The model under review builds one solid part; all positions refer to its coordinate system, in mm. A direction names the side the tool comes from. Round coordinates to 2 decimals unless told otherwise and drop trailing zeros. Loops run counter-clockwise (first coordinate to the right, second up) from the corner with the lowest first, then second, coordinate; pieces in that order, holes last. Notation, with made-up numbers: M 3,35 L 12,35 A27 ccw 12,70 Z; hole C 20.25,53.25 d10. An arc over 180 degrees is marked long. Answer as a JSON object with one key per item and string values. Group by question number.
Item 1: Tool access review of faces 1 (the face through (0, -15, -20)), 2 (the face through (-10, 8, -15)): name each direction out of +Z, -Z, +X, -X, +Y, -Y from which nothing blocks a thin tool from reaching the whole face with its end or side.
Item 2: Insertion check: P1, Ø1.5, axis at x = -1, z = -9, coming from the +Y side. The pin has a flat end and moves straight along its axis. Give the tip position at first contact, or say it passes through.
Item 3: Consider section A-A (x = 23). Give the boundary of the cut face in (y, z).
Item 4: To check wall thickness, follow line 1 (Z direction, x = 2, y = 5); line 2 (Y direction, x = 9, z = -14.75); line 3 (X direction, y = 2, z = -26.75). State the ranges of each line that lie inside material, in increasing order.
Item 5: The part is to be moulded in two halves that separate along Z. For faces 3 (the face through (-28, -30.63, -28.57)), 4 (the face through (5.27, 4, -14.79)), 5 (the face through (23, -15, -24)), say which applies: +Z half, -Z half, draft (parallel to the pull), parting line (faces both ways), or undercut.
```python
from build123d import *

# Parameters (mm, degrees)
SKETCH1_W           = 59
SKETCH1_H           = 30
BOSS_EXTRUDE1_DEPTH = 30
SKETCH2_R           = 2.5
SKETCH2_R_2         = 3.5
CUT_EXTRUDE1_DEPTH  = 52.674461778
SKETCH3_W           = 59
SKETCH3_H           = 60
BOSS_EXTRUDE2_DEPTH = 30
FILLET1_R           = 5
FILLET2_R           = 5
FILLET3_R           = 5
FILLET4_R           = 5


with BuildPart() as part:
    # Sketch1 → Boss-Extrude1 (new body)
    with BuildSketch(Plane.XY):
        Rectangle(SKETCH1_W, SKETCH1_H)
        Polygon((4, 2.727207794), (6.572792206, 5.3), (8, 5.3), (8, 3.1), (10, 5.1), (10, 10), (5.1, 10), (3.1, 8), (5.3, 8), (5.3, 6.572792206), (2.727207794, 4), (-2.727207794, 4), (-5.3, 6.572792206), (-5.3, 8), (-3.1, 8), (-5.1, 10), (-10, 10), (-10, 5.1), (-8, 3.1), (-8, 5.3), (-6.572792206, 5.3), (-4, 2.727207794), (-4, -2.727207794), (-6.572792206, -5.3), (-8, -5.3), (-8, -3.1), (-10, -5.1), (-10, -10), (-5.1, -10), (-3.1, -8), (-5.3, -8), (-5.3, -6.572792206), (-2.727207794, -4), (2.727207794, -4), (5.3, -6.572792206), (5.3, -8), (3.1, -8), (5.1, -10), (10, -10), (10, -5.1), (8, -3.1), (8, -5.3), (6.572792206, -5.3), (4, -2.727207794), align=None, mode=Mode.SUBTRACT)
    extrude(amount=-BOSS_EXTRUDE1_DEPTH)

    # Sketch2 → Cut-Extrude1 (cut, through all)
    with BuildSketch(Plane(origin=(0, 15, 0), x_dir=(1, 0, 0), z_dir=(0, 1, 0))):
        with Locations(Location((0, 10, 0), (0, 0, 270))):
            Circle(SKETCH2_R)
        with Locations(Location((0, 20, 0), (0, 0, 270))):
            Circle(SKETCH2_R)
        with Locations(Location((-23, 24.5, 0), (0, 0, 270))):
            Circle(SKETCH2_R_2)
        with Locations(Location((23, 24.5, 0), (0, 0, 270))):
            Circle(SKETCH2_R_2)
        with Locations(Location((23, 11.5, 0), (0, 0, 270))):
            Circle(SKETCH2_R_2)
        with Locations(Location((-23, 11.5, 0), (0, 0, 270))):
            Circle(SKETCH2_R_2)
    extrude(amount=-CUT_EXTRUDE1_DEPTH, mode=Mode.SUBTRACT)

    # Sketch3 → Boss-Extrude2 (add)
    with BuildSketch(Plane.XY):
        with Locations((0, -45)):
            Rectangle(SKETCH3_W, SKETCH3_H)
    extrude(amount=-BOSS_EXTRUDE2_DEPTH)

    # Fillet1
    fillet1_edges = [part.edges().sort_by_distance(p)[0] for p in [
        (29.5, -30, 0),
    ]]
    fillet(fillet1_edges, radius=FILLET1_R)

    # Fillet2
    fillet2_edges = [part.edges().sort_by_distance(p)[0] for p in [
        (29.5, -30, -30),
    ]]
    fillet(fillet2_edges, radius=FILLET2_R)

    # Fillet3
    fillet3_edges = [part.edges().sort_by_distance(p)[0] for p in [
        (-29.5, -30, -30),
    ]]
    fillet(fillet3_edges, radius=FILLET3_R)

    # Fillet4
    fillet4_edges = [part.edges().sort_by_distance(p)[0] for p in [
        (-29.5, -30, 0),
    ]]
    fillet(fillet4_edges, radius=FILLET4_R)


solid = part.part
```
Geometry results:
{
 "1": {"face 1": "+Y", "face 2": "+Z, -Z"},
 "2": {"P1": "stops at y = -15"},
 "3": {"outline": "M -75,-30 L 15,-30 L 15,-28 L -15,-28 L -15,-21 L 15,-21 L 15,-15 L -15,-15 L -15,-8 L 15,-8 L 15,0 L -75,0 Z"},
 "4": {"line 1": "z = -30 to -21.5, -18.5 to -11.5, -8.5 to 0", "line 2": "y = -75 to -10, -4.1 to 4.1, 10 to 15", "line 3": "x = -29.18 to -25.68, -20.32 to -4, 4 to 20.32, 25.68 to 29.18"},
 "5": {"face 3": "-Z half", "face 4": "draft", "face 5": "undercut"}
}
